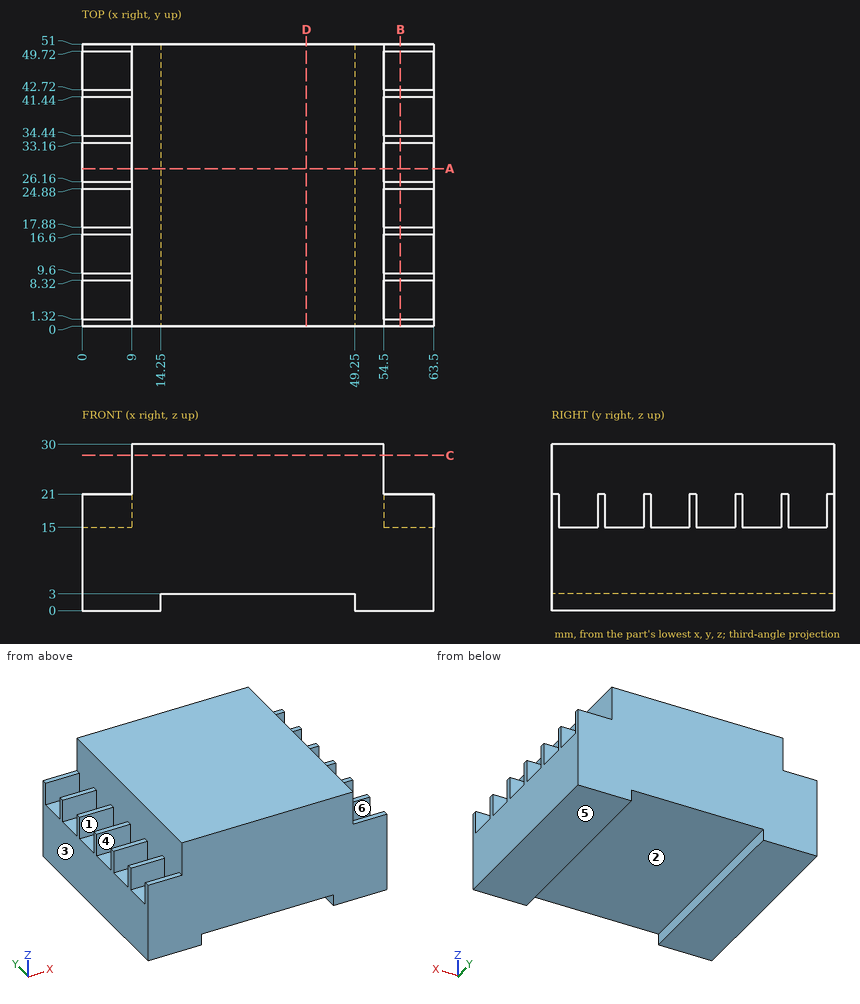
Check sheet for the drawn part. Datum: minimum x, y, z corner. Units: mm. A direction names the side the tool comes from. Round coordinates to 2 decimals unless told otherwise and drop trailing zeros. Loops run counter-clockwise (first coordinate to the right, second up) from the corner with the lowest first, then second, coordinate; pieces in that order, holes last. Notation, with made-up numbers: (24, 54.5) - (49, 54.5) arc R17 ccw to (49, 87.5) - close; hole circle Ø11 at (50.5, -9). An arc over 180 degrees is marked (long way). Write item = value, one per line. Start each with the question number.
1. Section check A-A on y = 28.5. Enter the section's corners in (x, z), then the cut area to 3 significant figures.
2. Set-up check for the marked faces 4, 5 and 6: record each of +Z, -Z, +X, -X, +Y, -Y from which the full face is reachable in a straight line by a thin tool's end or side.
3. Section check B-B on x = 57.5. Enter the section's corners in (y, z).
4. Depth check by flat-ended pin: pin 1 (1.1 mm diameter, centred on x = 4, y = 1, fed in from +Z); pin 2 (3.5 mm diameter, centred on x = 3.5, y = 31, fed in from +Z). Enter the tip coordinate at first touch or a pass-through.
5. Thickness scan on line 1 (X direction, y = 47, z = 27.5); line 2 (Z direction, x = 33, y = 48.5); line 3 (Z direction, x = 7.5, y = 36). Record the ranges inside material, lowest first.
6. Mould release check, pull along X, two halves, no side actions. Record for the marked faces 1, 2 and 3: released by +X, released by -X, zero draft, split by the parting line, or undercut.
7. Section check C-C on z = 28. Enter the section's corners in (x, y).
8. Section check D-D on x = 40.5. Enter the section's corners in (y, z), then the cut area to 3 significant figures.
Working result:
q1.outline = (0, 0) - (14.25, 0) - (14.25, 3) - (49.25, 3) - (49.25, 0) - (63.5, 0) - (63.5, 15) - (54.5, 15) - (54.5, 30) - (9, 30) - (9, 15) - (0, 15) - close
q1.area = 1,530 mm^2
q2.face_4 = +Z, -X
q2.face_5 = -Z, +X, -X, +Y, -Y
q2.face_6 = +Z, +X
q3.outline = (0, 0) - (51, 0) - (51, 21) - (49.72, 21) - (49.72, 15) - (42.72, 15) - (42.72, 21) - (41.44, 21) - (41.44, 15) - (34.44, 15) - (34.44, 21) - (33.16, 21) - (33.16, 15) - (26.16, 15) - (26.16, 21) - (24.88, 21) - (24.88, 15) - (17.88, 15) - (17.88, 21) - (16.6, 21) - (16.6, 15) - (9.6, 15) - (9.6, 21) - (8.32, 21) - (8.32, 15) - (1.32, 15) - (1.32, 21) - (0, 21) - close
q4.pin_1 = 21
q4.pin_2 = 15
q5.line_1 = 9 to 54.5
q5.line_2 = 3 to 30
q5.line_3 = 0 to 15
q6.face_1 = zero draft
q6.face_2 = undercut
q6.face_3 = released by -X
q7.outline = (9, 0) - (54.5, 0) - (54.5, 51) - (9, 51) - close
q8.outline = (0, 3) - (51, 3) - (51, 30) - (0, 30) - close
q8.area = 1,380 mm^2
